```python
from build123d import *

# Parameters (mm, degrees)
SKETCH1_R           = 5.08
BOSS_EXTRUDE1_DEPTH = 12.7
BOSS_EXTRUDE5_START = 2.54
SKETCH3_R           = 5.08
BOSS_EXTRUDE5_DEPTH = 2.54
BOSS_EXTRUDE7_DEPTH = 16.51
SKETCH6_R           = 3.897142563
BOSS_EXTRUDE8_DEPTH = 2.54


with BuildPart() as part:
    # Sketch1 → Boss-Extrude1 (new body)
    with BuildSketch(Plane.XY):
        Circle(SKETCH1_R)
        with BuildLine():
            Line((-1.27, 2.199704526), (-1.27, 3.81))
            Line((-1.27, 3.81), (1.27, 3.81))
            Line((1.27, 3.81), (1.27, 2.199704526))
            ThreePointArc((1.27, 2.199704526), (2.199704526, 1.27), (2.54, 0))
            ThreePointArc((2.54, 0), (-1.27, -2.199704526), (-1.27, 2.199704526))
        make_face(mode=Mode.SUBTRACT)
    extrude(amount=BOSS_EXTRUDE1_DEPTH)

    # Sketch3 → Boss-Extrude5 (add)
    with BuildSketch(Plane(origin=(0, 0, 0), x_dir=(-1, 0, 0), z_dir=(0, 0, -1)).offset(BOSS_EXTRUDE5_START)):
        Circle(SKETCH3_R)
    extrude(amount=-BOSS_EXTRUDE5_DEPTH)

    # Sketch5 → Boss-Extrude7 (add)
    with BuildSketch(Plane(origin=(0, 0, -2.54), x_dir=(-1, 0, 0), z_dir=(0, 0, -1))):
        with BuildLine():
            Line((-1.27, 5.715), (1.27, 5.715))
            Line((1.27, 5.715), (1.27, 2.909935566))
            ThreePointArc((1.27, 2.909935566), (0, -3.175), (-1.27, 2.909935566))
            Line((-1.27, 2.909935566), (-1.27, 5.715))
        make_face()
    extrude(amount=BOSS_EXTRUDE7_DEPTH)

    # Sketch6 → Boss-Extrude8 (add)
    with BuildSketch(Plane(origin=(0, 0, -19.05), x_dir=(-1, 0, 0), z_dir=(0, 0, -1))):
        with Locations(Location((0, 0, 0), (0, 0, 109.018885315))):
            Circle(SKETCH6_R)
    extrude(amount=BOSS_EXTRUDE8_DEPTH)


solid = part.part
```
Can you work these out from the model? Positions are in its coordinate system, mm. A direction names the side the tool comes from. Give positions to 0.01 mm unless a question says otherwise; leave off trailing zeros. Write each loop counter-clockwise with the first axis right and the second up, starting at its lowest first coordinate (ties: lowest second). Pieces come first, ordered by that corner, then holes. Notation, with made-up numbers: (58, 78.5) - (62, 78.5) arc R5 ccw to (62, 86.5) - close; hole circle Ø9 at (84.25, 51.5). An arc over 180 degrees is marked (long way). Write item = value, one per line. Start each with the question number.
1. For pin 1 (4 mm diameter, centred on y = 1.5, z = -14, fed in from +X) (3 decimals); pin 2 (6 mm diameter, centred on x = -4, z = 8.5, fed in from -Y); pin 3 (1.5 mm diameter, centred on x = 4, z = 7, fed in from -Y), each with a flat end and sliding along its axis, tell me the tip position at first contact or that it passes through.
2. Thinking about a two-plate mould opening in Z: for faces 1 (the face through (0.07, -3.34, -2.54)), 2 (the face through (-1.27, 3, 6)), 3 (the face through (-0.121, -3.173, -10.679)), 4 (the face through (0, 5, -19.05)), which applies, released by +Z, released by -Z, zero draft, split by the parting line, or undercut?
3. Imagine slicing it at D-D (y = 4.25). Please give me the cut outline in (x, z), and give its area (3 significant figures).
4. On a 3-axis mill with a long thin cutter (end or side, diameter ignored), from which of +Z, -Z, +X, -X, +Y, -Y can I reach the whole of each face in a straight line? I mean faces 5 (the face through (-1.27, 4, -11)), 6 (the face through (1.27, 4, -11)), 7 (the face through (-1.107, -3.737, -20.302)), 8 (the face through (0, 3.81, 6)), 9 (the face through (-2, -3, -19.05)). Say none if no direction works.
5. Imagine slicing it at A-A (x = 0). Please give me the cut outline in (y, z) (3 decimals), and give its area (3 significant figures).
6. Imagine slicing it at C-C (z = -7.5). Please give me the cut outline in (x, y) (3 decimals).
7. Please list where these lines run through material, in increasing order: line 1 (Z direction, x = -1.75, y = 2.75); line 2 (Y direction, x = 0, z = 5.5); line 3 (Z direction, x = 0.5, y = 2).
8. Imagine slicing it at B-B (y = 1.25). Please give me the cut outline in (x, z), and give its area (3 significant figures).
Worked answers:
q1.pin_1 = 3.175
q1.pin_2 = -4.98
q1.pin_3 = -3.9
q2.face_1 = undercut
q2.face_2 = zero draft
q2.face_3 = undercut
q2.face_4 = released by -Z
q3.outline = (-2.78, -2.54) - (-1.27, -2.54) - (-1.27, -19.05) - (1.27, -19.05) - (1.27, -2.54) - (2.78, -2.54) - (2.78, 12.7) - (-2.78, 12.7) - close
q3.area = 127 mm2
q4.face_5 = -X, +Y
q4.face_6 = +X, +Y
q4.face_7 = -Z
q4.face_8 = +Z
q4.face_9 = none
q5.outline = (-5.08, -2.54) - (-3.175, -2.54) - (-3.175, -19.05) - (-3.897, -19.05) - (-3.897, -21.59) - (3.897, -21.59) - (3.897, -19.05) - (5.715, -19.05) - (5.715, -2.54) - (5.08, -2.54) - (5.08, 12.7) - (3.81, 12.7) - (3.81, 0) - (-2.54, 0) - (-2.54, 12.7) - (-5.08, 12.7) - close
q5.area = 241 mm2
q6.outline = (-1.27, 2.91) arc R3.175 ccw (long way) to (1.27, 2.91) - (1.27, 5.715) - (-1.27, 5.715) - close
q7.line_1 = -21.59 to -19.05, -2.54 to 12.7
q7.line_2 = -5.08 to -2.54, 3.81 to 5.08
q7.line_3 = -21.59 to 0
q8.outline = (-4.92, -2.54) - (-2.92, -2.54) - (-2.92, -19.05) - (-3.69, -19.05) - (-3.69, -21.59) - (3.69, -21.59) - (3.69, -19.05) - (2.92, -19.05) - (2.92, -2.54) - (4.92, -2.54) - (4.92, 12.7) - (2.21, 12.7) - (2.21, 0) - (-2.21, 0) - (-2.21, 12.7) - (-4.92, 12.7) - close
q8.area = 209 mm2
